```python
from build123d import *

# Parameters (mm, degrees)
BOSS_EXTRUDE1_DEPTH     = 25
SKETCH2_W               = 4
SKETCH2_H               = 3
BOSS_EXTRUDE2_DEPTH     = 5
CUT_EXTRUDE1_DEPTH      = 26.670995306
CUT_EXTRUDE1_DEPTH_BACK = 26.670995306
SKETCH3_R               = 1.05


with BuildPart() as part:
    # Sketch1 → Boss-Extrude1 (new body)
    with BuildSketch(Plane(origin=(0, 0, 0), x_dir=(0, 0, -1), z_dir=(1, 0, 0))):
        Polygon((0, 0), (-5, 0), (-5, -3), align=None)
    extrude(amount=BOSS_EXTRUDE1_DEPTH)

    # Sketch2 → Boss-Extrude2 (add)
    with BuildSketch(Plane.XY.offset(5)):
        with Locations((12.5, -1.5)):
            Rectangle(SKETCH2_W, SKETCH2_H)
    extrude(amount=-BOSS_EXTRUDE2_DEPTH)

    # Sketch3 → Cut-Extrude1 (cut, two sides: drawn at the far end of the back side and taken through both)
    with BuildSketch(Plane(origin=(0, 0, 0), x_dir=(-1, 0, 0), z_dir=(0, 0, -1)).offset(-CUT_EXTRUDE1_DEPTH_BACK)):
        with Locations((-12.5, -1.5)):
            Circle(SKETCH3_R)
    extrude(amount=CUT_EXTRUDE1_DEPTH + CUT_EXTRUDE1_DEPTH_BACK, mode=Mode.SUBTRACT)


solid = part.part
```
Work out the finished part from the listing and answer in its coordinate system (mm). A direction names the side the tool comes from. Round coordinates to 2 decimals unless told otherwise and drop trailing zeros. Write each loop counter-clockwise with the first axis right and the second up, starting at its lowest first coordinate (ties: lowest second). Pieces come first, ordered by that corner, then holes.
1) Determine the mould class of faces 4 (the face through (25, -1, 3)), 5 (the face through (19.7, -1.5, 2.5)), 6 (the face through (11.5, -1.18, 2.54)) for opening direction X: pulls with the +X half, pulls with the -X half, needs draft (parallel to the pull), parting line crosses it, or undercut.
2) Consider probe 1 along Y at (x, z) = (12.5, 1.95); probe 2 along X at (y, z) = (-1.5, 3.6); probe 3 along X at (y, z) = (-1.5, 1.9). Determine where each line is inside the solid, lowest interval first.
3) A cutting plane is placed at C-C on x = 12.5. Determine the outline of the cut face in (y, z).
4) A cutting plane is placed at B-B on z = 4.3. Determine the outline of the cut face in (x, y).
5) A cutting plane is placed at D-D on z = 1.9. Determine the outline of the cut face in (x, y).
6) Which of the six approach directions +Z, -Z, +X, -X, +Y, -Y give full straight-line access (tool end or side, diameter ignored) to faces 1 (the face through (14.5, -2, 1)), 2 (the face through (12, 0, 2)), 3 (the face through (5.2, -1.5, 2.5))?
7) A cutting plane is placed at A-A on y = -1.5. Determine the outline of the cut face in (x, z).
Entries:
1. face 4: pulls with the +X half
1. face 5: needs draft
1. face 6: undercut
2. probe 1: y = -3 to -2.55, -0.45 to 0
2. probe 2: x = 0 to 11.45, 13.55 to 25
2. probe 3: x = 10.5 to 11.45, 13.55 to 14.5
3. outline: (-3, 0) - (-2.55, 0) - (-2.55, 5) - (-3, 5) - close; (-0.45, 0) - (0, 0) - (0, 5) - (-0.45, 5) - close
4. outline: (0, -2.58) - (10.5, -2.58) - (10.5, -3) - (14.5, -3) - (14.5, -2.58) - (25, -2.58) - (25, 0) - (0, 0) - close; hole circle Ø2.1 at (12.5, -1.5)
5. outline: (0, -1.14) - (10.5, -1.14) - (10.5, -3) - (14.5, -3) - (14.5, -1.14) - (25, -1.14) - (25, 0) - (0, 0) - close; hole circle Ø2.1 at (12.5, -1.5)
6. face 1: -Z, +X, -Y
6. face 2: +Z, -Z, +X, -X, +Y
6. face 3: -Z, -X, -Y
7. outline: (0, 2.5) - (10.5, 2.5) - (10.5, 0) - (11.45, 0) - (11.45, 5) - (0, 5) - close; (13.55, 0) - (14.5, 0) - (14.5, 2.5) - (25, 2.5) - (25, 5) - (13.55, 5) - close
